The drawing under review shows one solid part. Ordinate dimensions are in mm from its lowest x, y, z. Give positions to 0.01 mm unless a question says otherwise; leave off trailing zeros. Loops run counter-clockwise (first coordinate to the right, second up) from the corner with the lowest first, then second, coordinate; pieces in that order, holes last. Notation, with made-up numbers: (15, 81) -> (52, 81) arc R11 ccw to (52, 102) -> close; hole circle Ø4 at (72.5, 47.25). An arc over 180 degrees is marked (long way). Answer in a Markdown table with one row per item. Add a question column.
(1) For line 1 (X direction, y = 1.95, z = 5); line 2 (X direction, y = 2.3, z = 35); line 3 (X direction, y = 0.4, z = 6), list the stretches that pass through material, from the lowest coordinate up.
(2) Consider section B-B on z = 35. Write out the cut boundary in (x, y), then the cut area to 3 significant figures.
(3) Consider section C-C on z = 5. Write out the cut boundary in (x, y), then the cut area to 3 significant figures.
(4) Consider section A-A on x = 60. Write out the cut boundary in (y, z), then the cut area to 3 significant figures.
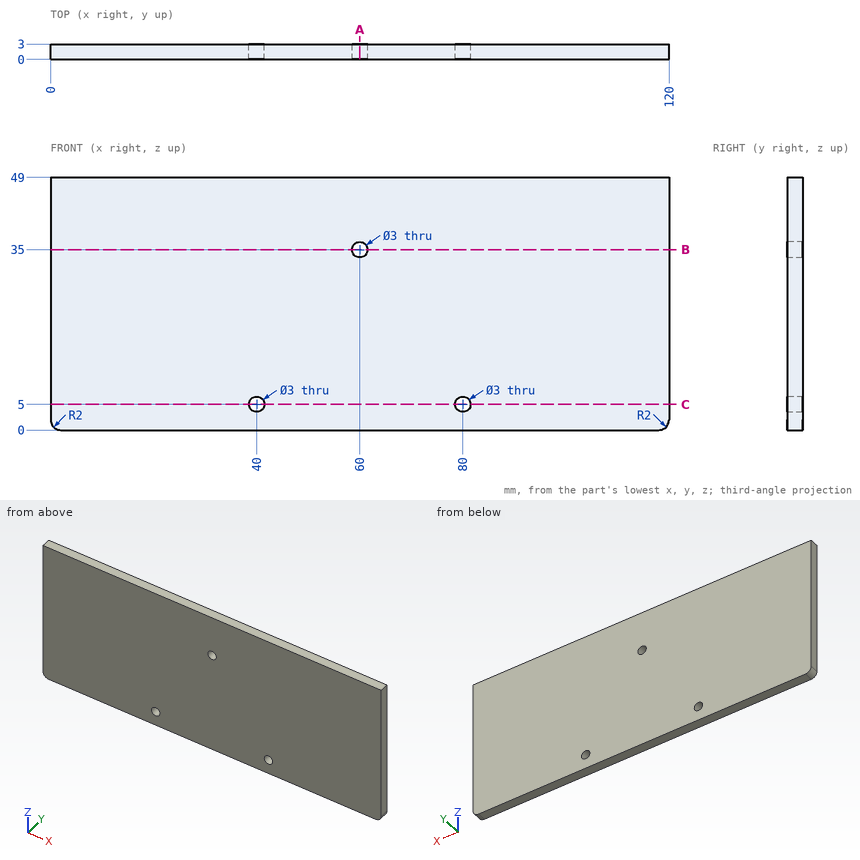
Values follow:
| question | item | result |
|---|---|---|
| 1 | line 1 | 0 to 38.5, 41.5 to 78.5, 81.5 to 120 |
| 1 | line 2 | 0 to 58.5, 61.5 to 120 |
| 1 | line 3 | 0 to 38.88, 41.12 to 78.88, 81.12 to 120 |
| 2 | outline | (0, 0) -> (58.5, 0) -> (58.5, 3) -> (0, 3) -> close; (61.5, 0) -> (120, 0) -> (120, 3) -> (61.5, 3) -> close |
| 2 | area | 351 mm2 |
| 3 | outline | (0, 0) -> (38.5, 0) -> (38.5, 3) -> (0, 3) -> close; (41.5, 0) -> (78.5, 0) -> (78.5, 3) -> (41.5, 3) -> close; (81.5, 0) -> (120, 0) -> (120, 3) -> (81.5, 3) -> close |
| 3 | area | 342 mm2 |
| 4 | outline | (0, 0) -> (3, 0) -> (3, 33.5) -> (0, 33.5) -> close; (0, 36.5) -> (3, 36.5) -> (3, 49) -> (0, 49) -> close |
| 4 | area | 138 mm2 |
